The figure shows three views and two pictorial views of one solid part (mm, origin at its lowest corner). Answer the questions. A direction names the side the tool comes from. Give positions to 0.01 mm unless a question says otherwise; leave off trailing zeros. Write each loop counter-clockwise with the first axis right and the second up, starting at its lowest first coordinate (ties: lowest second). Pieces come first, ordered by that corner, then holes. Notation, with made-up numbers: (89.5, 40) -> (131.5, 40) arc R23 ccw to (131.5, 78) -> close; hole circle Ø11 at (32.5, 71). An arc over 180 degrees is marked (long way). Write each question's results on one line, items separated by ' | '. Start each with the question number.
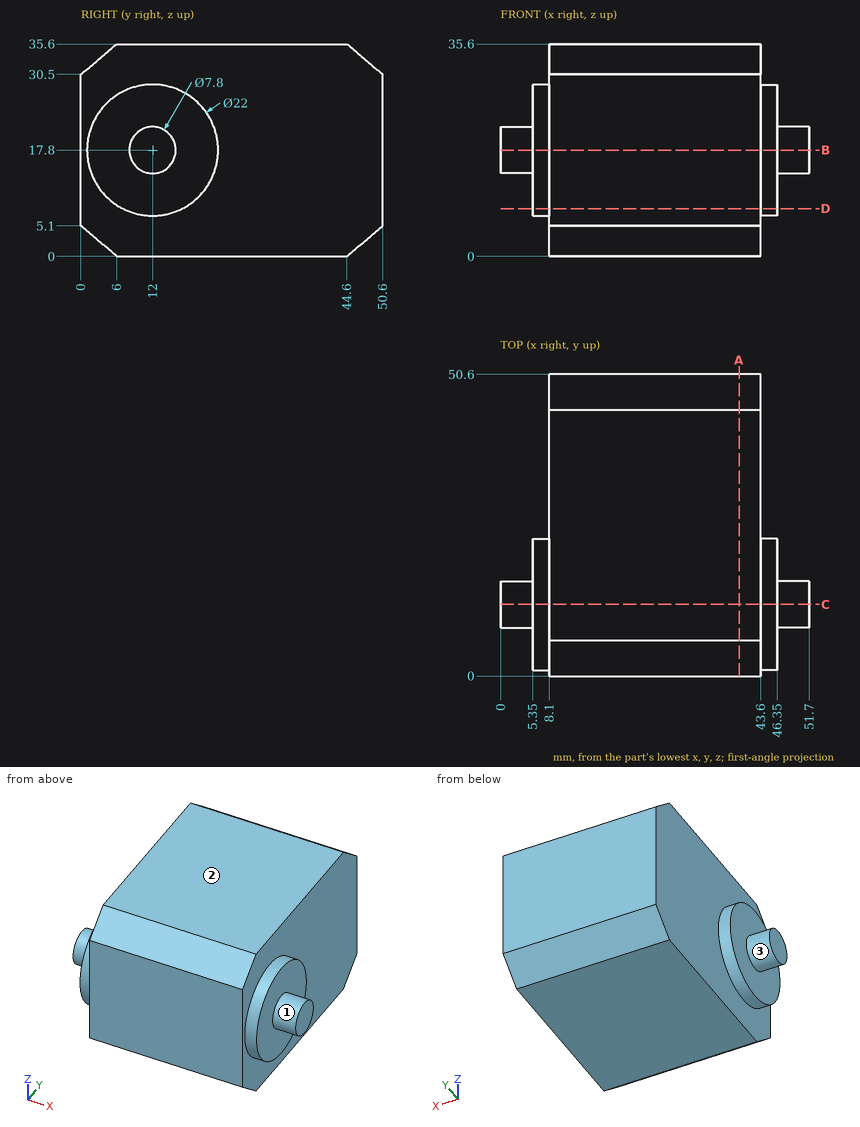
1. Section D-D (z = 8) is taken. Write down the section's boundary in (x, y), then the cut area to 3 significant figures.
2. Consider probe 1 along X at (y, z) = (29, 10.5); probe 2 along X at (y, z) = (13, 10.5); probe 3 along Y at (x, z) = (14.5, 33.5). Determine where each line is inside the solid, lowest interval first. Write a range as [from, to].
3. Section A-A (x = 40) is taken. Write down the section's boundary in (y, z), then the cut area to 3 significant figures.
4. Section B-B (z = 17.8) is taken. Write down the section's boundary in (x, y).
5. This flat-tipped pin is pushed along its axis until it touches: pin 1 Ø3 at (y, z) = (39, 11.5) entering from +X. Where does it stop, or does it pass through?
6. A tool of negligible diameter and unlimited length cuts with its end or side. For the marked faces 1, 2 and 3, from which of +Z, -Z, +X, -X, +Y, -Y can it reach the whole face along a straight path? Write none if from no direction.
7. Section C-C (y = 12) is taken. Write down the section's boundary in (x, z), then the cut area to 3 significant figures.
Results:
1) outline: (5.35, 7) -> (8.1, 7) -> (8.1, 0) -> (43.6, 0) -> (43.6, 7) -> (46.35, 7) -> (46.35, 17) -> (43.6, 17) -> (43.6, 50.6) -> (8.1, 50.6) -> (8.1, 17) -> (5.35, 17) -> close | area: 1,850 mm²
2) probe 1: x = [8.1, 43.6] | probe 2: x = [5.35, 46.35] | probe 3: y = [3.53, 47.07]
3) outline: (0, 5.1) -> (6, 0) -> (44.6, 0) -> (50.6, 5.1) -> (50.6, 30.5) -> (44.6, 35.6) -> (6, 35.6) -> (0, 30.5) -> close | area: 1,740 mm²
4) outline: (0, 8.1) -> (5.35, 8.1) -> (5.35, 1) -> (8.1, 1) -> (8.1, 0) -> (43.6, 0) -> (43.6, 1) -> (46.35, 1) -> (46.35, 8.1) -> (51.7, 8.1) -> (51.7, 15.9) -> (46.35, 15.9) -> (46.35, 23) -> (43.6, 23) -> (43.6, 50.6) -> (8.1, 50.6) -> (8.1, 23) -> (5.35, 23) -> (5.35, 15.9) -> (0, 15.9) -> close
5) pin 1: stops at x = 43.6
6) face 1: +X | face 2: +Z, +X, -X, +Y, -Y | face 3: -X
7) outline: (0, 13.9) -> (5.35, 13.9) -> (5.35, 6.8) -> (8.1, 6.8) -> (8.1, 0) -> (43.6, 0) -> (43.6, 6.8) -> (46.35, 6.8) -> (46.35, 13.9) -> (51.7, 13.9) -> (51.7, 21.7) -> (46.35, 21.7) -> (46.35, 28.8) -> (43.6, 28.8) -> (43.6, 35.6) -> (8.1, 35.6) -> (8.1, 28.8) -> (5.35, 28.8) -> (5.35, 21.7) -> (0, 21.7) -> close | area: 1,470 mm²
